from build123d import *

# Parameters (mm, degrees)
SKETCH1_W           = 75
SKETCH1_H           = 35
SKETCH1_R           = 2.35
SKETCH1_W_2         = 40.5
SKETCH1_H_2         = 20
BOSS_EXTRUDE1_DEPTH = 4


with BuildPart() as part:
    # Sketch1 → Boss-Extrude1 (new body)
    with BuildSketch(Plane.XY):
        Rectangle(SKETCH1_W, SKETCH1_H)
        with Locations((-24.55, 4.85)):
            Circle(SKETCH1_R, mode=Mode.SUBTRACT)
        with Locations((-24.55, -4.85)):
            Circle(SKETCH1_R, mode=Mode.SUBTRACT)
        with Locations((24.55, -4.85)):
            Circle(SKETCH1_R, mode=Mode.SUBTRACT)
        with Locations((24.55, 4.85)):
            Circle(SKETCH1_R, mode=Mode.SUBTRACT)
        Rectangle(SKETCH1_W_2, SKETCH1_H_2, mode=Mode.SUBTRACT)
    extrude(amount=BOSS_EXTRUDE1_DEPTH)


solid = part.part
Input: part model. Units: mm. Frame: model coordinates. A direction names the side the tool comes from. Give positions to 0.01 mm unless a question says otherwise; leave off trailing zeros. Loops run counter-clockwise (first coordinate to the right, second up) from the corner with the lowest first, then second, coordinate; pieces in that order, holes last. Notation, with made-up numbers: M -6,-25 L 3,-25 A21 ccw 3,-17 Z; hole C 71,58.25 d3. An arc over 180 degrees is marked long. Use one line per item in the form item = value.
1. Section query D-D, the plane z = 2.15. Return the cut outline in (x, y).
Numbers:
outline = M -37.5,-17.5 L 37.5,-17.5 L 37.5,17.5 L -37.5,17.5 Z; hole C -24.55,-4.85 d4.7; hole C -24.55,4.85 d4.7; hole M -20.25,-10 L 20.25,-10 L 20.25,10 L -20.25,10 Z; hole C 24.55,-4.85 d4.7; hole C 24.55,4.85 d4.7
2. Line query: L1, parallel to Y at x = 24.55, z = 1.75; L2, parallel to X at y = 5, z = 1.4; L3, parallel to Y at x = 14.5, z = 2.5. Output: solid intervals per line, ascending.
Numbers:
L1 = -17.5 to -7.2, -2.5 to 2.5, 7.2 to 17.5
L2 = -37.5 to -26.9, -22.2 to -20.25, 20.25 to 22.2, 26.9 to 37.5
L3 = -17.5 to -10, 10 to 17.5
3. Section query C-C, the plane x = 5. Return the cut outline in (y, z).
Numbers:
outline = M -17.5,0 L -10,0 L -10,4 L -17.5,4 Z; M 10,0 L 17.5,0 L 17.5,4 L 10,4 Z
4. Section query B-B, the plane y = -4.85. Return the cut outline in (x, z), and give its area (3 significant figures).
Numbers:
outline = M -37.5,0 L -26.9,0 L -26.9,4 L -37.5,4 Z; M -22.2,0 L -20.25,0 L -20.25,4 L -22.2,4 Z; M 20.25,0 L 22.2,0 L 22.2,4 L 20.25,4 Z; M 26.9,0 L 37.5,0 L 37.5,4 L 26.9,4 Z
area = 100 mm²
5. Pull-direction query (Y, two-part tool) for faces 1 (the face through (22.202, -4.747, 1.972)), 2 (the face through (-1, 17.5, 2)), 3 (the face through (-1, -17.5, 2)), 4 (the face through (37.5, 0, 2)); classes: released by +Y, released by -Y, zero draft, split by the parting line, or undercut.
Numbers:
face_1 = undercut
face_2 = released by +Y
face_3 = released by -Y
face_4 = zero draft
6. Reachability of faces 5 (the face through (-1, 12, 0)), 6 (the face through (-20.25, 0, 2)) from +Z, -Z, +X, -X, +Y, -Y: full face, straight path, thin tool, end or side. Return the list, or none.
Numbers:
face_5 = -Z, +X, -X, +Y, -Y
face_6 = +Z, -Z
7. Section query A-A, the plane x = -24.55. Return the cut outline in (y, z), and give its area (3 significant figures).
Numbers:
outline = M -17.5,0 L -7.2,0 L -7.2,4 L -17.5,4 Z; M -2.5,0 L 2.5,0 L 2.5,4 L -2.5,4 Z; M 7.2,0 L 17.5,0 L 17.5,4 L 7.2,4 Z
area = 102 mm²
